Source: CAD feature listing. Evaluate the final solid. Frame: model axes, mm. Face numbers are marked on the shaded views. A direction names the side the tool comes from. Give positions to 0.01 mm unless a question says otherwise; leave off trailing zeros. Order: outer loops, then holes, each group sorted by start corner. A loop starts at its lowest first (then second) coordinate and runs counter-clockwise, first axis right, second up. Notation, with made-up numbers: M 17.5,-5 L 36.5,-5 A15 cw 36.5,10 Z; hole C 44,-8 d4. An arc over 180 degrees is marked long. Use CSV: the item, a comma, the result in double quotes. Start each with the question number.
Item 1: Section query C-C on x = 10. Return loops of the section in (y, z).
Item 2: Access query for the marked faces 1, 2 and 3. Directions: +Z, -Z, +X, -X, +Y, -Y. A direction counts if a zero-diameter tool reaches every point of the face in a straight line with its end or side. Return the directions, or none.
Item 3: Section query D-D on z = -19. Return loops of the section in (x, y).
Item 4: Section query A-A on z = 3.5. Return loops of the section in (x, y).
Item 5: Ray query, probe 1 along X at (y, z) = (8.5, -4); probe 2 along Z at (x, y) = (22.5, 1.75). Return the intervals inside material, ascending. Write a range as from..to.
Item 6: First-contact query: pin 1 (4 mm diameter, centred on x = 72.5, z = 17.5, fed in from +Y); pin 2 (3 mm diameter, centred on y = 5.5, z = 8, fed in from -X); pin 3 (5 mm diameter, centred on x = 44, y = 1, fed in from +Z); pin 4 (12 mm diameter, centred on x = -33.5, z = -17, fed in from -Y). Flat tips, straight axial feed; report the tip coordinate or a pass-through.
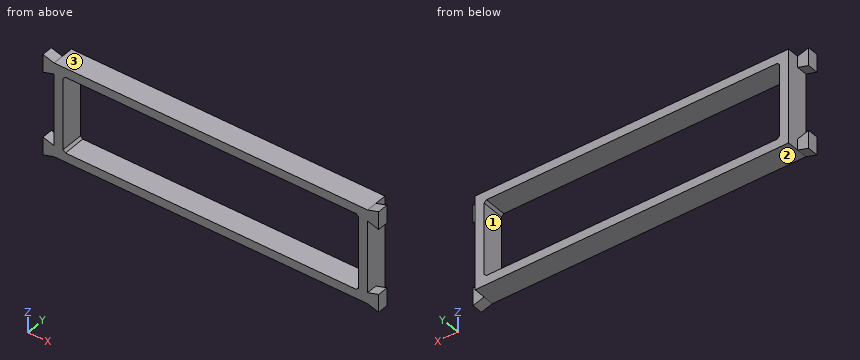
from build123d import *

# Parameters (mm, degrees)
SKETCH1_W           = 138.3
SKETCH1_H           = 41.58498921
BOSS_EXTRUDE1_DEPTH = 10
BOSS_EXTRUDE2_DEPTH = 4.8


with BuildPart() as part:
    # Sketch1 → Boss-Extrude1 (new body)
    with BuildSketch(Plane(origin=(0, 0, 0), x_dir=(1, 0, 0), z_dir=(0, 1, 0))):
        Rectangle(SKETCH1_W, SKETCH1_H)
        Polygon((-64.15, 16.792494605), (64.15, 16.792494605), (65.15, 15.792494605), (65.15, -15.792494605), (64.15, -16.792494605), (-64.15, -16.792494605), (-65.15, -15.792494605), (-65.15, 15.792494605), align=None, mode=Mode.SUBTRACT)
    extrude(amount=BOSS_EXTRUDE1_DEPTH)

    # Sketch3 → Boss-Extrude2 (add)
    with BuildSketch(Plane.XZ):
        Polygon((74.05, 22.283333333), (69.15, 20.783333333), (69.15, 15.883333333), (74.05, 14.383333333), align=None)
        Polygon((74.05, -14.383333333), (69.15, -15.883333333), (69.15, -20.783333333), (74.05, -22.283333333), align=None)
        Polygon((-74.05, 22.283333333), (-69.15, 20.783333333), (-69.15, 15.883333333), (-74.05, 14.383333333), align=None)
        Polygon((-74.05, -14.383333333), (-69.15, -15.883333333), (-69.15, -20.783333333), (-74.05, -22.283333333), align=None)
    extrude(amount=-BOSS_EXTRUDE2_DEPTH)


solid = part.part
Verdict:
1,outline,"M 0,-20.79 L 10,-20.79 L 10,-16.79 L 0,-16.79 Z; M 0,16.79 L 10,16.79 L 10,20.79 L 0,20.79 Z"
2,face 1,"+Y, -Y"
2,face 2,"-Z, +Y, -Y"
2,face 3,"+Z, +Y, -Y"
3,outline,"M -74.05,0 L 74.05,0 L 74.05,4.8 L 69.15,4.8 L 69.15,10 L -69.15,10 L -69.15,4.8 L -74.05,4.8 Z"
4,outline,"M -69.15,0 L -65.15,0 L -65.15,10 L -69.15,10 Z; M 65.15,0 L 69.15,0 L 69.15,10 L 65.15,10 Z"
5,probe 1,"-69.15..-65.15, 65.15..69.15"
5,probe 2,"-20.79..-16.79, 16.79..20.79"
6,pin 1,"y = 4.8"
6,pin 2,"x = -69.15"
6,pin 3,"z = 20.79"
6,pin 4,"y = 0"
